from build123d import *

# Parameters (mm, degrees)
ESBO_O1_R                = 50
RESSALTO_EXTRUS_O1_DEPTH = 2
ESBO_O2_R                = 2.75
CORTE_EXTRUS_O1_DEPTH    = 2
ESBO_O3_R                = 1.75
ESBO_O3_R_2              = 1.27
CORTE_EXTRUS_O2_DEPTH    = 10


with BuildPart() as part:
    # Esboço1 → Ressalto-extrusão1 (new body)
    with BuildSketch(Plane.XY):
        Circle(ESBO_O1_R)
    extrude(amount=RESSALTO_EXTRUS_O1_DEPTH)

    # Esboço2 → Corte-extrusão1 (cut)
    with BuildSketch(Plane.XY.offset(2)):
        with Locations((-29, -34.409301068)):
            Circle(ESBO_O2_R)
        with Locations((29, -34.409301068)):
            Circle(ESBO_O2_R)
        with Locations((-38.824197531, 22.752619324)):
            Circle(ESBO_O2_R)
        with Locations((38.824197531, 22.752619324)):
            Circle(ESBO_O2_R)
    extrude(amount=-CORTE_EXTRUS_O1_DEPTH, mode=Mode.SUBTRACT)

    # Esboço3 → Corte-extrusão2 (cut)
    with BuildSketch(Plane.XY.offset(2)):
        with Locations((-25.1, 14.54)):
            Circle(ESBO_O3_R)
        with Locations((24.33, -15.91)):
            Circle(ESBO_O3_R)
        with Locations((-39.88, -12.25)):
            Circle(ESBO_O3_R)
        with Locations((-39.88, 12.25)):
            Circle(ESBO_O3_R)
        with Locations((39.88, 12.25)):
            Circle(ESBO_O3_R)
        with Locations((39.88, -12.25)):
            Circle(ESBO_O3_R)
        with Locations((6.79, 27.4)):
            Circle(ESBO_O3_R_2)
        with Locations((22.03, 27.4)):
            Circle(ESBO_O3_R_2)
        with Locations((-8.21, -28.46)):
            Circle(ESBO_O3_R_2)
        with Locations((-23.45, -28.46)):
            Circle(ESBO_O3_R_2)
    extrude(amount=-CORTE_EXTRUS_O2_DEPTH, mode=Mode.SUBTRACT)


solid = part.part
Could you check a few things on this model? Use its own coordinates, in mm. Round coordinates to 2 decimals unless told otherwise and drop trailing zeros. Loops run counter-clockwise (first coordinate to the right, second up) from the corner with the lowest first, then second, coordinate; pieces in that order, holes last. Notation, with made-up numbers: (57, -18.5) -> (109, -18.5) arc R19 cw to (109, 14.5) -> close; hole circle Ø6 at (64.25, -12). An arc over 180 degrees is marked (long way). Use CSV: the item, a comma, the result in double quotes.
(1) Suppose I cut it at D-D on y = -28.46. Write out the boundary of the cut face in (x, z), plus the area to 3 significant figures.
Return value:
outline,"(-41.11, 0) -> (-24.72, 0) -> (-24.72, 2) -> (-41.11, 2) -> close; (-22.18, 0) -> (-9.48, 0) -> (-9.48, 2) -> (-22.18, 2) -> close; (-6.94, 0) -> (41.11, 0) -> (41.11, 2) -> (-6.94, 2) -> close"
area,"154 mm²"
(2) Suppose I cut it at C-C on z = 1.25. Give the number of separate pieces and of enclosed holes in the cut face, plus the area to 3 significant figures.
Return value:
separate pieces,"1"
enclosed holes,"14"
area,"7,680 mm²"
(3) Will these pins go through, and if not, where does the flat tip stop? pin 1 Ø2 at (x, y) = (-23.45, -28.46) entering from +Z; pin 2 Ø6 at (x, y) = (-2.5, -6.5) entering from -Z; pin 3 Ø1 at (x, z) = (-31.5, 1) entering from +Y.
Return value:
pin 1,"passes through"
pin 2,"stops at z = 0"
pin 3,"stops at y = 39.23"
(4) Suppose I cut it at B-B on x = 29. Write out the boundary of the cut face in (y, z), plus the area to 3 significant figures.
Return value:
outline,"(-40.73, 0) -> (-37.16, 0) -> (-37.16, 2) -> (-40.73, 2) -> close; (-31.66, 0) -> (40.73, 0) -> (40.73, 2) -> (-31.66, 2) -> close"
area,"152 mm²"
(5) If I drill on probe 1 along X at (y, z) = (21, 0.1); probe 2 along X at (y, z) = (-13.5, 1.3); probe 3 along Y at (x, z) = (29.5, 0.1), over which ranges is the centre line in solid material (lowest first)? Write a range as [from, to].
Return value:
probe 1,"x = [-45.38, -40.94], [-36.71, 36.71], [40.94, 45.38]"
probe 2,"x = [-48.14, -41.1], [-38.66, 38.66], [41.1, 48.14]"
probe 3,"y = [-40.37, -37.11], [-31.71, 40.37]"
(6) If we mould it in two halves opening along Y, with no side actions, what happens to faces 1 (the flat face through (-1, 1, 2)), 2 (the cylindrical face through (25.999, -15.384, 1.014)), 3 (the cylindrical face through (47.69, 15.02, 0.99))? For each: +Y half, -Y half, draft (parallel to the pull), parting line (faces both ways), or undercut.
Return value:
face 1,"draft"
face 2,"undercut"
face 3,"parting line"
(7) Suppose I cut it at A-A on y = 27.4. Write out the boundary of the cut face in (x, z), plus the area to 3 significant figures.
Return value:
outline,"(-41.82, 0) -> (5.52, 0) -> (5.52, 2) -> (-41.82, 2) -> close; (8.06, 0) -> (20.76, 0) -> (20.76, 2) -> (8.06, 2) -> close; (23.3, 0) -> (41.82, 0) -> (41.82, 2) -> (23.3, 2) -> close"
area,"157 mm²"
